Input: part model. Units: mm. Frame: model coordinates. A direction names the side the tool comes from. Give positions to 0.01 mm unless a question says otherwise; leave off trailing zeros. Write each loop counter-clockwise with the first axis right and the second up, starting at its lowest first coordinate (ties: lowest second). Pieces come first, ordered by that corner, then holes. Notation, with made-up numbers: (47, -31) - (58, -31) arc R7 ccw to (58, -21) - close; hole circle Ø2 at (-4.5, 29). An arc over 180 degrees is marked (long way). Use a Markdown table: item, result. Add a question column.
1. Set-up query: faces 1 (the cylindrical face through (0.28, 0.162, 26.842)), 2 (the flat face through (0, -1, -55)), 3 (the flat face through (0, 1, -57)). Return all of +Z, -Z, +X, -X, +Y, -Y with unobstructed straight access to the full face (end or side cutting, diameter ignored); none if empty.
2. Section query C-C, the plane y = 2.5. Return loops of the section in (x, z).
3. Material intervals for probe 1 along Y at (x, z) = (-0.5, -21.5); probe 2 along Z at (x, y) = (-17.5, -1.5); probe 3 along Z at (x, y) = (10.5, 3.5), sorted ascending.
4. Section query A-A, the plane x = -5. Return loops of the section in (y, z), plus the area to 3 significant figures.
5. Pin query (flat end, axial travel): pin 1 (10 mm diameter, centred on x = -15, z = -53.5, fed in from -Y); pin 2 (4 mm diameter, centred on x = -13, z = -70.5, fed in from +Y); pin 3 (2.5 mm diameter, centred on y = 0, z = 22.85, fed in from +X). Return the tip coordinate at first contact, or that it passes through.
6. Section query B-B, the plane z = -94. Return loops of the section in (x, y), plus the area to 3 significant figures.
```python
from build123d import *

# Parameters (mm, degrees)
SKETCH1_R                = 4
SKETCH1_R_2              = 1
BOSS_EXTRUDE1_DEPTH      = 20
BOSS_EXTRUDE1_DEPTH_BACK = 20


with BuildPart() as part:
    # Sketch1 → Boss-Extrude1 (new body, two sides)
    with BuildSketch(Plane(origin=(0, 0, 0), x_dir=(0, 0, -1), z_dir=(1, 0, 0))) as boss_extrude1_sk:
        with Locations((-22.845337752, 0)):
            Circle(SKETCH1_R)
        with Locations((-22.845337752, 0)):
            Circle(SKETCH1_R_2, mode=Mode.SUBTRACT)
        with BuildLine():
            Line((131.027645594, 1), (-18.972354406, 1))
            ThreePointArc((-18.972354406, 1), (-18.877218967, 0.50401717), (-18.845337752, 0))
            ThreePointArc((-18.845337752, 0), (-18.877218967, -0.50401717), (-18.972354406, -1))
            Line((-18.972354406, -1), (131.027645594, -1))
            Line((131.027645594, -1), (131.027645594, 1))
        make_face()
    extrude(amount=BOSS_EXTRUDE1_DEPTH)
    extrude(boss_extrude1_sk.sketch, amount=-BOSS_EXTRUDE1_DEPTH_BACK)


solid = part.part
```
Result sheet:
| question | item | result |
|---|---|---|
| 1 | face 1 | +X, -X |
| 1 | face 2 | -Z, +X, -X, -Y |
| 1 | face 3 | -Z, +X, -X, +Y |
| 2 | outline | (-20, 19.72) - (20, 19.72) - (20, 25.97) - (-20, 25.97) - close |
| 3 | probe 1 | y = -1 to 1 |
| 3 | probe 2 | z = 19.14 to 26.55 |
| 3 | probe 3 | z = 20.91 to 24.78 |
| 4 | outline | (-1, -131.03) - (1, -131.03) - (1, 18.97) arc R4 ccw (long way) to (-1, 18.97) - close; hole circle Ø2 at (0, 22.85) |
| 4 | area | 347 mm² |
| 5 | pin 1 | stops at y = -1 |
| 5 | pin 2 | stops at y = 1 |
| 5 | pin 3 | stops at x = 20 |
| 6 | outline | (-20, -1) - (20, -1) - (20, 1) - (-20, 1) - close |
| 6 | area | 80.0 mm² |
